```python
from build123d import *

# Parameters (mm, degrees)
BOSS_EXTRUDE1_DEPTH = 10
SKETCH6_W           = 128.025007892
SKETCH6_H           = 8
BOSS_EXTRUDE3_DEPTH = 10


with BuildPart() as part:
    # Sketch1 → Boss-Extrude1 (new body)
    with BuildSketch(Plane(origin=(0, 0, 0), x_dir=(1, 0, 0), z_dir=(0, 1, 0))):
        Polygon((0, 0), (-128.025007892, 22.574263097), (-128.025007892, 52.574263097), (-139.025007892, 52.574263097), (-139.025007892, 62.574263097), (-128.025007892, 62.574263097), (0, 40), (0, 10), (11, 10), (11, 0), align=None)
    extrude(amount=BOSS_EXTRUDE1_DEPTH)

    # Sketch6 → Boss-Extrude3 (add)
    with BuildSketch(Plane.XZ):
        with Locations((-64.012503946, -30.7)):
            Rectangle(SKETCH6_W, SKETCH6_H)
    extrude(amount=BOSS_EXTRUDE3_DEPTH)


solid = part.part
```
Could you check a few things on this model? Use its own coordinates, in mm. A direction names the side the tool comes from. Coordinates: 2 decimals unless noted, no trailing zeros. Loops run counter-clockwise (first coordinate to the right, second up) from the corner with the lowest first, then second, coordinate; pieces in that order, holes last. Notation, with made-up numbers: M 68,21 L 96,21 A31 ccw 96,59 Z; hole C 18,-34.5 d2. An arc over 180 degrees is marked long. Put each result on its own line as item: value. Start each with the question number.
(1) I need wall thicknesses on line 1 (Y direction, x = -119, z = -46); line 2 (Z direction, x = -80, y = -1.75); line 3 (Z direction, x = -15.5, y = 7). Which ranges of each line are inside material? Lowest first, please. Write a range as from..to.
(2) Suppose I cut it at A-A on y = 6. Please give me the cut outline in (x, z) (3 decimals).
(3) Suppose I cut it at C-C on z = -5. Please give me the cut outline in (x, y).
(4) For faces 1 (the face through (-65, -5, -34.7)), 2 (the face through (-133, 5, -52.574)), 3 (the face through (-65, -5, -26.7)), 4 (the face through (5, 5, -10)), which set-ups out of +Z, -Z, +X, -X, +Y, -Y let a thin tool reach every point of the face, with its end or its side?
(5) Suppose I cut it at D-D on y = -5. Please give me the cut outline in (x, z) (3 decimals), then the cut area to 3 significant figures.
(6) Will these pins go through, and if not, where does the flat tip stop? P1, Ø5, axis at x = -74.5, y = 7.5, coming from the +Z side; P2, Ø8, axis at x = -38, y = -3.5, coming from the -Z side; P3, Ø1, axis at x = -74.5, y = -7, coming from the +Z side; P4, Ø12, axis at x = -115, z = -9.5, coming from the -Y side.
(7) Suppose I cut it at B-B on x = -63.5. Please give me the cut outline in (y, z), then the cut area to 3 significant figures.
Solutions:
1. line 1: y = 0..10
1. line 2: z = -34.7..-26.7
1. line 3: z = -42.73..-2.73
2. outline: M -139.025,-62.574 L -128.025,-62.574 L 0,-40 L 0,-10 L 11,-10 L 11,0 L 0,0 L -128.025,-22.574 L -128.025,-52.574 L -139.025,-52.574 Z
3. outline: M -28.36,0 L 11,0 L 11,10 L -28.36,10 Z
4. face 1: -Z, +X, -X, -Y
4. face 2: +Z, -X, +Y, -Y
4. face 3: +Z, +X, -X, -Y
4. face 4: -Z, +X, +Y, -Y
5. outline: M -128.025,-34.7 L 0,-34.7 L 0,-26.7 L -128.025,-26.7 Z
5. area: 1,020 mm2
6. P1: stops at z = -12.7
6. P2: stops at z = -47.04
6. P3: stops at z = -26.7
6. P4: passes through
7. outline: M -10,-34.7 L 0,-34.7 L 0,-51.2 L 10,-51.2 L 10,-11.2 L 0,-11.2 L 0,-26.7 L -10,-26.7 Z
7. area: 480 mm2
